from build123d import *

# Parameters (mm, degrees)
BOSS_EXTRUDE1_DEPTH = 6.35
CUT_EXTRUDE1_DEPTH  = 319.315227787
SKETCH3_W           = 6.35
SKETCH3_H           = 12.7
CUT_EXTRUDE2_DEPTH  = 319.315227787
SKETCH4_W           = 58.894470958
SKETCH4_H           = 80.433020337
BOSS_EXTRUDE3_DEPTH = 6.35
SKETCH6_W           = 17.78
SKETCH6_H           = 27.94
CUT_EXTRUDE3_DEPTH  = 319.315227787
CUT_EXTRUDE4_DEPTH  = 6.35


with BuildPart() as part:
    # Sketch1 → Boss-Extrude1 (new body)
    with BuildSketch(Plane.XY):
        with BuildLine():
            Line((133.35, 0), (135.457692, 0))
            Line((135.457692, 0), (135.457692, 287.9852))
            Line((135.457692, 287.9852), (25.4, 287.9852))
            ThreePointArc((25.4, 287.9852), (7.439487758, 280.545712242), (0, 262.5852))
            Line((0, 262.5852), (0, 0))
            Line((0, 0), (0, -6.35))
            Line((0, -6.35), (19.05, -6.35))
            Line((19.05, -6.35), (19.05, 0))
            Line((19.05, 0), (38.1, 0))
            Line((38.1, 0), (38.1, -6.35))
            Line((38.1, -6.35), (57.15, -6.35))
            Line((57.15, -6.35), (57.15, 0))
            Line((57.15, 0), (76.2, 0))
            Line((76.2, 0), (76.2, -6.35))
            Line((76.2, -6.35), (95.25, -6.35))
            Line((95.25, -6.35), (95.25, 0))
            Line((95.25, 0), (114.3, 0))
            Line((114.3, 0), (114.3, -6.35))
            Line((114.3, -6.35), (133.35, -6.35))
            Line((133.35, -6.35), (133.35, 0))
        make_face()
    extrude(amount=BOSS_EXTRUDE1_DEPTH)

    # Sketch2 → Cut-Extrude1 (cut, through all)
    with BuildSketch(Plane.XY.offset(6.35)):
        with BuildLine():
            Line((73.66, 22.86), (73.66, 78.74))
            ThreePointArc((73.66, 78.74), (76.635795103, 85.924204897), (83.82, 88.9))
            Line((83.82, 88.9), (114.3, 88.9))
            ThreePointArc((114.3, 88.9), (121.484204897, 85.924204897), (124.46, 78.74))
            Line((124.46, 78.74), (124.46, 22.86))
            ThreePointArc((124.46, 22.86), (121.484204897, 15.675795103), (114.3, 12.7))
            Line((114.3, 12.7), (83.82, 12.7))
            ThreePointArc((83.82, 12.7), (76.635795103, 15.675795103), (73.66, 22.86))
        make_face()
        with BuildLine():
            Line((20.32, 12.7), (50.8, 12.7))
            ThreePointArc((50.8, 12.7), (57.984204897, 15.675795103), (60.96, 22.86))
            Line((60.96, 22.86), (60.96, 78.74))
            ThreePointArc((60.96, 78.74), (57.984204897, 85.924204897), (50.8, 88.9))
            Line((50.8, 88.9), (20.32, 88.9))
            ThreePointArc((20.32, 88.9), (13.135795103, 85.924204897), (10.16, 78.74))
            Line((10.16, 78.74), (10.16, 22.86))
            ThreePointArc((10.16, 22.86), (13.135795103, 15.675795103), (20.32, 12.7))
        make_face()
        with BuildLine():
            Line((73.66, 196.85), (73.66, 265.43))
            ThreePointArc((73.66, 265.43), (75.519871939, 269.920128061), (80.01, 271.78))
            Line((80.01, 271.78), (118.11, 271.78))
            ThreePointArc((118.11, 271.78), (122.600128061, 269.920128061), (124.46, 265.43))
            Line((124.46, 265.43), (124.46, 196.85))
            ThreePointArc((124.46, 196.85), (122.600128061, 192.359871939), (118.11, 190.5))
            Line((118.11, 190.5), (80.01, 190.5))
            ThreePointArc((80.01, 190.5), (75.519871939, 192.359871939), (73.66, 196.85))
        make_face()
        with BuildLine():
            Line((10.16, 196.85), (10.16, 265.43))
            ThreePointArc((10.16, 265.43), (12.019871939, 269.920128061), (16.51, 271.78))
            Line((16.51, 271.78), (54.61, 271.78))
            ThreePointArc((54.61, 271.78), (59.100128061, 269.920128061), (60.96, 265.43))
            Line((60.96, 265.43), (60.96, 196.85))
            ThreePointArc((60.96, 196.85), (59.100128061, 192.359871939), (54.61, 190.5))
            Line((54.61, 190.5), (16.51, 190.5))
            ThreePointArc((16.51, 190.5), (12.019871939, 192.359871939), (10.16, 196.85))
        make_face()
        with BuildLine():
            Line((73.66, 107.95), (73.66, 171.45))
            ThreePointArc((73.66, 171.45), (75.519871939, 175.940128061), (80.01, 177.8))
            Line((80.01, 177.8), (118.11, 177.8))
            ThreePointArc((118.11, 177.8), (122.600128061, 175.940128061), (124.46, 171.45))
            Line((124.46, 171.45), (124.46, 107.95))
            ThreePointArc((124.46, 107.95), (122.600128061, 103.459871939), (118.11, 101.6))
            Line((118.11, 101.6), (80.01, 101.6))
            ThreePointArc((80.01, 101.6), (75.519871939, 103.459871939), (73.66, 107.95))
        make_face()
        with BuildLine():
            Line((10.16, 107.95), (10.16, 171.45))
            ThreePointArc((10.16, 171.45), (12.019871939, 175.940128061), (16.51, 177.8))
            Line((16.51, 177.8), (54.61, 177.8))
            ThreePointArc((54.61, 177.8), (59.100128061, 175.940128061), (60.96, 171.45))
            Line((60.96, 171.45), (60.96, 107.95))
            ThreePointArc((60.96, 107.95), (59.100128061, 103.459871939), (54.61, 101.6))
            Line((54.61, 101.6), (16.51, 101.6))
            ThreePointArc((16.51, 101.6), (12.019871939, 103.459871939), (10.16, 107.95))
        make_face()
    extrude(amount=-CUT_EXTRUDE1_DEPTH, mode=Mode.SUBTRACT)

    # Sketch3 → Cut-Extrude2 (cut, through all)
    with BuildSketch(Plane.XY.offset(6.35)):
        with Locations((3.175, 0)):
            Rectangle(SKETCH3_W, SKETCH3_H)
        with Locations((79.375, 0)):
            Rectangle(SKETCH3_W, SKETCH3_H)
    extrude(amount=-CUT_EXTRUDE2_DEPTH, mode=Mode.SUBTRACT)

    # Sketch4 → Boss-Extrude3 (add)
    with BuildSketch(Plane.XY.offset(6.35)):
        with Locations((98.603069985, 49.657450477)):
            Rectangle(SKETCH4_W, SKETCH4_H)
    extrude(amount=-BOSS_EXTRUDE3_DEPTH)

    # Sketch6 → Cut-Extrude3 (cut, through all)
    with BuildSketch(Plane(origin=(0, 0, 0), x_dir=(-1, 0, 0), z_dir=(0, 0, -1))):
        with Locations((-115.57, 74.93)):
            Rectangle(SKETCH6_W, SKETCH6_H)
    extrude(amount=-CUT_EXTRUDE3_DEPTH, mode=Mode.SUBTRACT)

    # Sketch7 → Cut-Extrude4 (cut)
    with BuildSketch(Plane.XY.offset(6.35)):
        with BuildLine():
            Line((82.55, 88.9), (86.868, 88.9))
            ThreePointArc((86.868, 88.9), (93.154179285, 86.296179285), (95.758, 80.01))
            Line((95.758, 80.01), (95.758, 21.59))
            ThreePointArc((95.758, 21.59), (93.154179285, 15.303820715), (86.868, 12.7))
            Line((86.868, 12.7), (82.55, 12.7))
            ThreePointArc((82.55, 12.7), (76.263820715, 15.303820715), (73.66, 21.59))
            Line((73.66, 21.59), (73.66, 80.01))
            ThreePointArc((73.66, 80.01), (76.263820715, 86.296179285), (82.55, 88.9))
        make_face()
    extrude(amount=-CUT_EXTRUDE4_DEPTH, mode=Mode.SUBTRACT)


solid = part.part
The model under review builds one solid part; all positions refer to its coordinate system, in mm. A direction names the side the tool comes from. Round coordinates to 2 decimals unless told otherwise and drop trailing zeros. Order: outer loops, then holes, each group sorted by start corner. A loop starts at its lowest first (then second) coordinate and runs counter-clockwise, first axis right, second up. Notation, with made-up numbers: (67.5, 41.25) -> (77.5, 41.25) arc R16 cw to (77.5, 62.25) -> close; hole circle Ø2 at (-17, 13). An arc over 180 degrees is marked (long way). Write item = value, one per line. Start each with the question number.
Item 1: Consider section B-B on x = 48. Write out the cut boundary in (y, z).
Item 2: For faces 1 (the face through (124.46, 232, 3)), 2 (the face through (38.1, -3, 3)), 3 (the face through (133.35, -3, 3)), 4 (the face through (67, 143, 0)), list the 3-axis set-ups (+Z, -Z, +X, -X, +Y, -Y) from which the entire face can be reached by the end or side of a thin tool; tool diameter is ignored.
Item 3: Consider section D-D on z = 1. Count the separate pieces of the cut face and the enclosed holes in it, plus the area to 3 significant figures.
Item 4: Consider section A-A on y = 219.5. Write out the cut boundary in (x, z), plus the area to 3 significant figures.
Item 5: For line 1 along X through (y, z) = (260.5, 5.75); line 2 along Y through (x, z) = (46, 5.25); line 3 along Y through (x, z) = (24, 2.25), list the stretches that pass through material, from the lowest coordinate up.
Item 6: Mouldability with a two-part tool opening along Y and no side actions: class faces 5 (the face through (10.16, 51, 3)), 6 (the face through (76.2, 3, 3)), 7 (the face through (81, 287.985, 3)) as released by +Y, released by -Y, zero draft, split by the parting line, or undercut.
Item 7: Consider section C-C on y = 86. Write out the cut boundary in (x, z), plus the area to 3 significant figures.
Conclusion:
q1.outline = (-6.35, 0) -> (12.7, 0) -> (12.7, 6.35) -> (-6.35, 6.35) -> close; (88.9, 0) -> (101.6, 0) -> (101.6, 6.35) -> (88.9, 6.35) -> close; (177.8, 0) -> (190.5, 0) -> (190.5, 6.35) -> (177.8, 6.35) -> close; (271.78, 0) -> (287.99, 0) -> (287.99, 6.35) -> (271.78, 6.35) -> close
q2.face_1 = +Z, -Z
q2.face_2 = +Z, -Z, -Y
q2.face_3 = +Z, -Z, +X, -Y
q2.face_4 = -Z, +X, -X, +Y, -Y
q3.separate_pieces = 1
q3.enclosed_holes = 7
q3.area = 17,400 mm2
q4.outline = (0, 0) -> (10.16, 0) -> (10.16, 6.35) -> (0, 6.35) -> close; (60.96, 0) -> (73.66, 0) -> (73.66, 6.35) -> (60.96, 6.35) -> close; (124.46, 0) -> (135.46, 0) -> (135.46, 6.35) -> (124.46, 6.35) -> close
q4.area = 215 mm2
q5.line_1 = 0 to 10.16, 60.96 to 73.66, 124.46 to 135.46
q5.line_2 = -6.35 to 12.7, 88.9 to 101.6, 177.8 to 190.5, 271.78 to 287.99
q5.line_3 = 0 to 12.7, 88.9 to 101.6, 177.8 to 190.5, 271.78 to 287.95
q6.face_5 = undercut
q6.face_6 = zero draft
q6.face_7 = released by +Y
q7.outline = (0, 0) -> (13.21, 0) -> (13.21, 6.35) -> (0, 6.35) -> close; (57.91, 0) -> (75.98, 0) -> (75.98, 6.35) -> (57.91, 6.35) -> close; (93.44, 0) -> (106.68, 0) -> (106.68, 6.35) -> (93.44, 6.35) -> close; (124.46, 0) -> (135.46, 0) -> (135.46, 6.35) -> (124.46, 6.35) -> close
q7.area = 353 mm2
